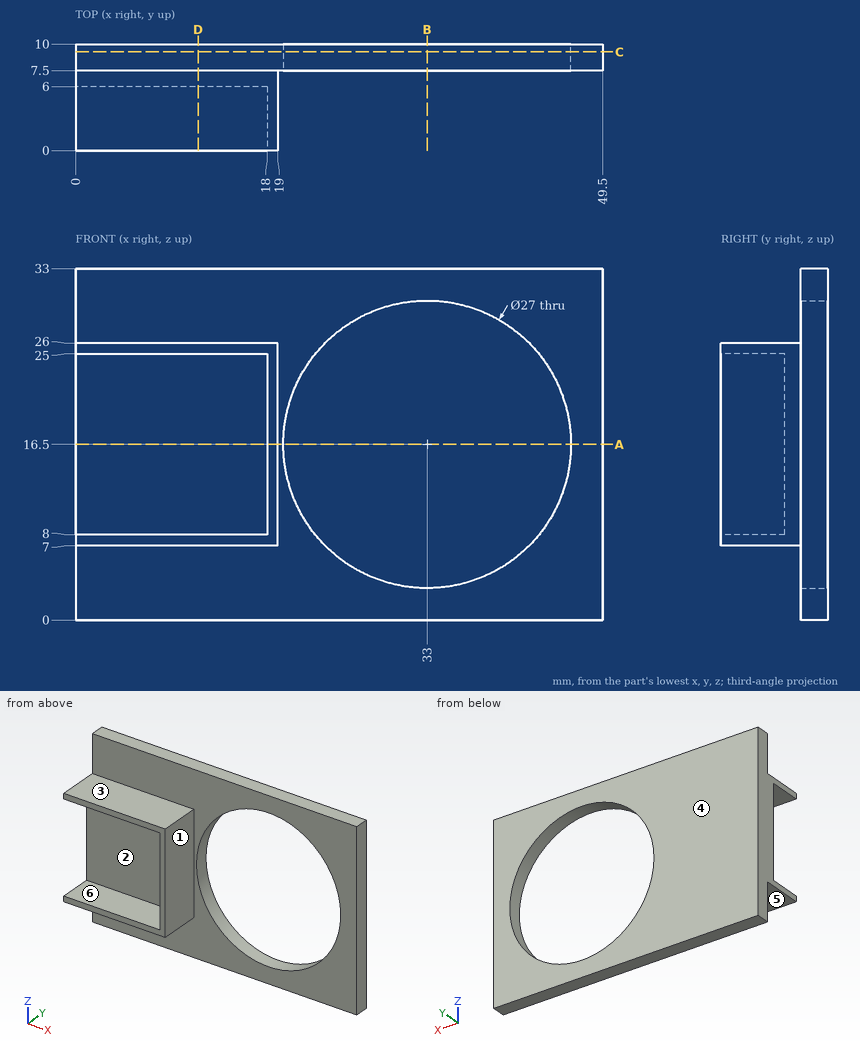
Geometry check sheet. Reference: drawing and pictorial views, mm from the part's lowest x, y, z. A direction names the side the tool comes from. Round coordinates to 2 decimals unless told otherwise and drop trailing zeros. Order: outer loops, then holes, each group sorted by start corner. A loop starts at its lowest first (then second) coordinate and runs counter-clockwise, first axis right, second up. Notation, with made-up numbers: (63.25, 25) - (87.25, 25) arc R25 ccw to (87.25, 41) - close; hole circle Ø5 at (-39, -33). An arc over 180 degrees is marked (long way). One line per question, with ' | ' between items. Start each with the question number.
(1) Access from +Z, -Z, +X, -X, +Y, -Y to the whole of each face (thin tool, end or side, straight path). Record for the marked faces 1, 2 and 3.
(2) Release check for a two-part mould opening along Z. For the marked faces 4, 5 and 6 record: released by +Z, released by -Z, zero draft, split by the parting line, or undercut.
(3) Thickness scan on L1, parallel to Z at x = 33, y = 8.15; L2, parallel to Z at x = 6.5, y = 0.75; L3, parallel to X at y = 4.25, z = 14.5. Record the ranges inside material, lowest first. Write a range as [from, to].
(4) Depth check by flat-ended pin: pin 1 Ø1 at (y, z) = (5.5, 25) entering from +X; pin 2 Ø3 at (x, y) = (6.5, 2) entering from -Z; pin 3 Ø1 at (y, z) = (4, 20) entering from -X. Enter the tip coordinate at first touch or a pass-through.
(5) Sectioned sample at D-D on x = 11.5. Record the cut outline in (y, z), and give its area (3 significant figures).
(6) Sectioned sample at A-A on z = 16.5. Record the cut outline in (x, y).
(7) Sectioned sample at B-B on x = 33. Record the cut outline in (y, z), and give its area (3 significant figures).
(8) Sectioned sample at C-C on y = 9.25. Record the cut outline in (x, z).
Conclusion:
1) face 1: +Z, -Z, +X, -Y | face 2: -X, -Y | face 3: +Z, +X, -X, -Y
2) face 4: zero draft | face 5: released by -Z | face 6: undercut
3) L1: z = [0, 3], [30, 33] | L2: z = [7, 8], [25, 26] | L3: x = [18, 19]
4) pin 1: stops at x = 19 | pin 2: stops at z = 7 | pin 3: stops at x = 18
5) outline: (0, 7) - (7.5, 7) - (7.5, 0) - (10, 0) - (10, 33) - (7.5, 33) - (7.5, 26) - (0, 26) - (0, 25) - (6, 25) - (6, 8) - (0, 8) - close | area: 123 mm2
6) outline: (0, 6) - (18, 6) - (18, 0) - (19, 0) - (19, 7.5) - (19.5, 7.5) - (19.5, 10) - (0, 10) - close; (46.5, 7.5) - (49.5, 7.5) - (49.5, 10) - (46.5, 10) - close
7) outline: (7.5, 0) - (10, 0) - (10, 3) - (7.5, 3) - close; (7.5, 30) - (10, 30) - (10, 33) - (7.5, 33) - close | area: 15.0 mm2
8) outline: (0, 0) - (49.5, 0) - (49.5, 33) - (0, 33) - close; hole circle Ø27 at (33, 16.5)
